```python
from build123d import *

# Parameters (mm, degrees)
STOCK_PLATE_BETA1_1_START       = 76.165904354
STOCK_PLATE_BETA1_1_OUTLINE_W   = 152.4
STOCK_PLATE_BETA1_1_OUTLINE_H   = 152.4
STOCK_PLATE_BETA1_1_OUTLINE_W_2 = 139.7
STOCK_PLATE_BETA1_1_OUTLINE_H_2 = 66.690053594
STOCK_PLATE_BETA1_1_OUTLINE_H_3 = 66.659946406
STOCK_PLATE_BETA1_1_DEPTH       = 6.384095646
STOCK_PLATE_BETA1_1_START_2     = 11.43
STOCK_PLATE_BETA1_1_2_OUTLINE_W = 6.35
STOCK_PLATE_BETA1_1_2_OUTLINE_H = 6.35
STOCK_PLATE_BETA1_1_2_DEPTH     = 64.735904354
SKETCH1_R                       = 1.59512
CUT_EXTRUDE2_DEPTH              = 8.89


# Read off the part's stored shape, not the designer's step: Stock-plate_beta1-1
with BuildPart() as part:
    # Stock-plate_beta1-1 outline → Stock-plate_beta1-1 (new body)
    with BuildSketch(Plane(origin=(0, 0, 0), x_dir=(1, 0, 0), z_dir=(0, 1, 0)).offset(STOCK_PLATE_BETA1_1_START)):
        with Locations((40.776583963, 45.362139437)):
            Rectangle(STOCK_PLATE_BETA1_1_OUTLINE_W, STOCK_PLATE_BETA1_1_OUTLINE_H)
        with Locations((40.776583963, 81.86711264)):
            Rectangle(STOCK_PLATE_BETA1_1_OUTLINE_W_2, STOCK_PLATE_BETA1_1_OUTLINE_H_2, mode=Mode.SUBTRACT)
        with Locations((40.776583963, 8.84211264)):
            Rectangle(STOCK_PLATE_BETA1_1_OUTLINE_W_2, STOCK_PLATE_BETA1_1_OUTLINE_H_3, mode=Mode.SUBTRACT)
    extrude(amount=STOCK_PLATE_BETA1_1_DEPTH)

    # Stock-plate_beta1-1 2 outline → Stock-plate_beta1-1 2 (add)
    with BuildSketch(Plane(origin=(0, 0, 0), x_dir=(1, 0, 0), z_dir=(0, 1, 0)).offset(STOCK_PLATE_BETA1_1_START_2)):
        with Locations((-32.248416037, 118.387139437)):
            Rectangle(STOCK_PLATE_BETA1_1_2_OUTLINE_W, STOCK_PLATE_BETA1_1_2_OUTLINE_H)
        with Locations((113.801583963, 118.387139437)):
            Rectangle(STOCK_PLATE_BETA1_1_2_OUTLINE_W, STOCK_PLATE_BETA1_1_2_OUTLINE_H)
        with Locations((-32.248416037, -27.662860563)):
            Rectangle(STOCK_PLATE_BETA1_1_2_OUTLINE_W, STOCK_PLATE_BETA1_1_2_OUTLINE_H)
        with Locations((113.801583963, -27.662860563)):
            Rectangle(STOCK_PLATE_BETA1_1_2_OUTLINE_W, STOCK_PLATE_BETA1_1_2_OUTLINE_H)
    extrude(amount=STOCK_PLATE_BETA1_1_2_DEPTH)

    # Sketch1 → Cut-Extrude2 (cut)
    with BuildSketch(Plane(origin=(0, 11.43, 0), x_dir=(-1, 0, 0), z_dir=(0, -1, 0))):
        with Locations(Location((32.248416037, -27.662860563, 0), (0, 0, 90))):
            Circle(SKETCH1_R)
        with Locations(Location((-113.801583963, -27.662860563, 0), (0, 0, 90))):
            Circle(SKETCH1_R)
        with Locations(Location((-113.801583963, 118.387139437, 0), (0, 0, 90))):
            Circle(SKETCH1_R)
        with Locations(Location((32.248416037, 118.387139437, 0), (0, 0, 90))):
            Circle(SKETCH1_R)
    extrude(amount=-CUT_EXTRUDE2_DEPTH, mode=Mode.SUBTRACT)


solid = part.part
```
Model file for the job. Use its own axes, mm. A direction names the side the tool comes from. Give positions to 0.01 mm unless a question says otherwise; leave off trailing zeros. Loops run counter-clockwise (first coordinate to the right, second up) from the corner with the lowest first, then second, coordinate; pieces in that order, holes last. Notation, with made-up numbers: M 80,-29 L 101,-29 A9 ccw 101,-18 Z; hole C 27.5,78 d10. An arc over 180 degrees is marked long. Use one line per item in the form item = value.
Item 1: Two-plate mould, pull along Z, no slides. Class faces 6 (the flat face through (110.627, 43, 28)), 7 (the flat face through (40, 78, 30.838)), 8 (the flat face through (40, 79, -115.212)): released by +Z, released by -Z, zero draft, split by the parting line, or undercut.
Filled in:
face_6 = zero draft
face_7 = released by +Z
face_8 = undercut
Item 2: Drill centre lines: L1, parallel to Z at x = 3, y = 76.5; L2, parallel to X at y = 79, z = -74. Where is each one in solid material? Low to high.
Filled in:
L1 = -121.56 to -115.21, -48.52 to -42.17, 24.49 to 30.84
L2 = -35.42 to -29.07, 110.63 to 116.98
Item 3: Which spindle directions (+Z, -Z, +X, -X, +Y, -Y) get a long thin tool onto all of the face, cutting with end or side? Do faces 1 (the flat face through (40, 76.166, 28)), 2 (the flat face through (116.977, 78, -45)), 3 (the flat face through (40, 82.55, -46)), 4 (the flat face through (-32, 43, 24.488)), 5 (the flat face through (-29.073, 79, -81)). Say none if no direction does.
Filled in:
face_1 = +Z, -Z, -Y
face_2 = +Z, -Z, +X, +Y, -Y
face_3 = +Z, -Z, +X, -X, +Y
face_4 = +X, -X, -Y
face_5 = +Y, -Y
Item 4: Slice it at C-C on x = 33. List the corners of the cut face in (y, z), and give its area (3 significant figures).
Filled in:
outline = M 76.17,-121.56 L 82.55,-121.56 L 82.55,-115.21 L 76.17,-115.21 Z; M 76.17,-48.52 L 82.55,-48.52 L 82.55,-42.17 L 76.17,-42.17 Z; M 76.17,24.49 L 82.55,24.49 L 82.55,30.84 L 76.17,30.84 Z
area = 122 mm^2
Item 5: Slice it at A-A on z = -67.5. List the corners of the cut face in (x, y), and give its area (3 significant figures).
Filled in:
outline = M -35.42,76.17 L -29.07,76.17 L -29.07,82.55 L -35.42,82.55 Z; M 110.63,76.17 L 116.98,76.17 L 116.98,82.55 L 110.63,82.55 Z
area = 81.1 mm^2
Item 6: Flat gauge pins, fed straight in: pin 1 Ø3.5 at (x, z) = (114, -119) entering from -Y; pin 2 Ø1 at (x, z) = (54.5, -50) entering from -Y; pin 3 Ø5 at (x, z) = (75, -119) entering from -Y. Where does each tip first touch, or does it go through?
Filled in:
pin_1 = 11.43
pin_2 = through
pin_3 = 76.17
Item 7: Slice it at B-B on y = 46.5. List the corners of the cut face in (x, z).
Filled in:
outline = M -35.42,-121.56 L -29.07,-121.56 L -29.07,-115.21 L -35.42,-115.21 Z; M -35.42,24.49 L -29.07,24.49 L -29.07,30.84 L -35.42,30.84 Z; M 110.63,-121.56 L 116.98,-121.56 L 116.98,-115.21 L 110.63,-115.21 Z; M 110.63,24.49 L 116.98,24.49 L 116.98,30.84 L 110.63,30.84 Z
